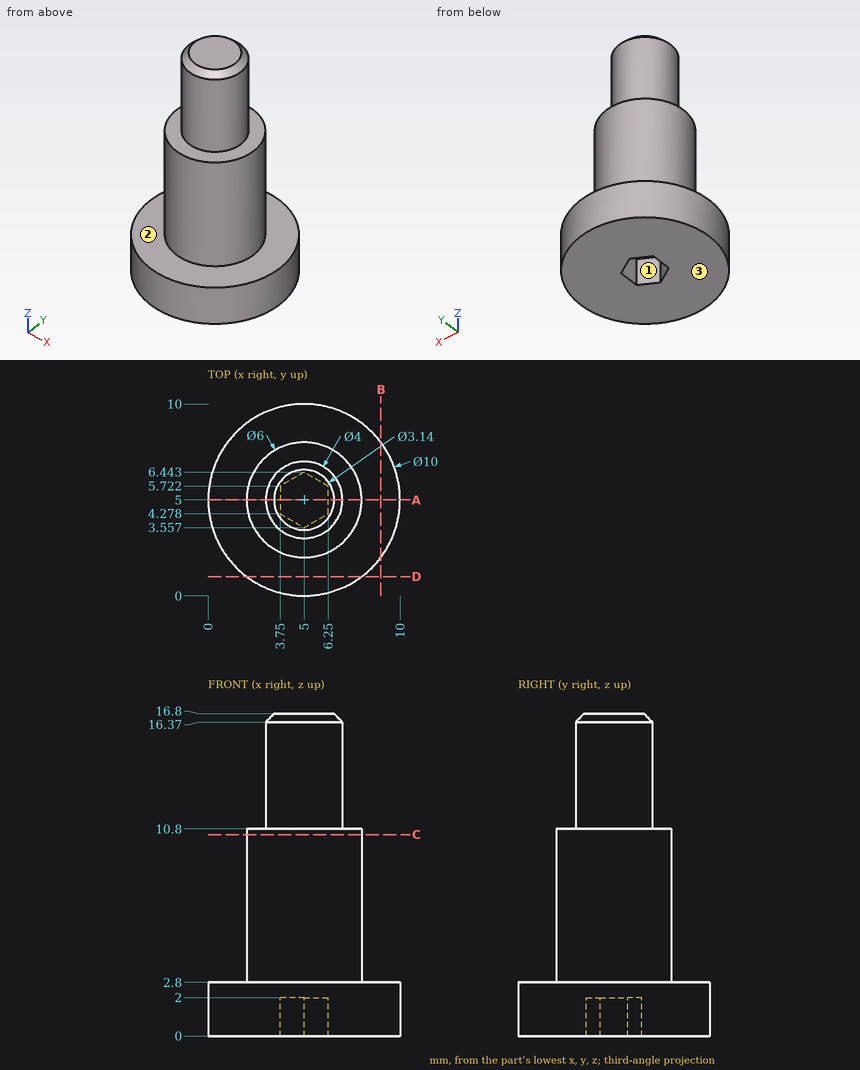
For this review, use the dimensioned drawing (mm, ordinates from the lowest corner) and the shaded views. A direction names the side the tool comes from. Coordinates: 2 decimals unless noted, no trailing zeros. Loops run counter-clockwise (first coordinate to the right, second up) from the corner with the lowest first, then second, coordinate; pieces in that order, holes last. Notation, with made-up numbers: (3.25, -23) -> (28.25, -23) arc R22 cw to (28.25, 3) -> close; hole circle Ø10 at (-40, 27.5). An arc over 180 degrees is marked (long way). Use a Markdown table: item, result. Add a question column.
1. Clearance check with flat-ended pins moving along their axes: pin 1 Ø1.2 at (y, z) = (4.5, 1) entering from +X; pin 2 Ø3 at (x, z) = (7.5, 4.5) entering from -Y; pin 3 Ø2 at (y, z) = (4, 6) entering from -X; pin 4 Ø3 at (x, z) = (7, 9.5) entering from +Y. State where each tip first meets the part, or that it passes through.
2. Add section C-C on z = 10.5. Write out the cut boundary in (x, y).
3. Add section A-A on y = 5. Write out the cut boundary in (x, z).
4. To check wall thickness, follow line 1 (Z direction, x = 1.75, y = 1.75); line 2 (Z direction, x = 5.5, y = 4); line 3 (Y direction, x = 6.75, z = 10) (1 decimal). State the ranges of each line that lie inside material, in increasing order.
5. Add section B-B on x = 9. Write out the cut boundary in (y, z).
6. Machinability: for the marked faces 1, 2 and 3, which of the approach directions +Z, -Z, +X, -X, +Y, -Y give a long, thin tool a straight path to every point of the face, cutting with its end or side? Answer none if there is none.
Returned:
| question | item | result |
|---|---|---|
| 1 | pin 1 | stops at x = 10 |
| 1 | pin 2 | stops at y = 2.17 |
| 1 | pin 3 | stops at x = 2 |
| 1 | pin 4 | stops at y = 7.96 |
| 2 | outline | circle Ø6 at (5, 5) |
| 3 | outline | (0, 0) -> (3.75, 0) -> (3.75, 2) -> (6.25, 2) -> (6.25, 0) -> (10, 0) -> (10, 2.8) -> (8, 2.8) -> (8, 10.8) -> (7, 10.8) -> (7, 16.37) -> (6.57, 16.8) -> (3.43, 16.8) -> (3, 16.37) -> (3, 10.8) -> (2, 10.8) -> (2, 2.8) -> (0, 2.8) -> close |
| 4 | line 1 | z = 0 to 2.8 |
| 4 | line 2 | z = 2 to 16.8 |
| 4 | line 3 | y = 2.6 to 7.4 |
| 5 | outline | (2, 0) -> (8, 0) -> (8, 2.8) -> (2, 2.8) -> close |
| 6 | face 1 | -Z |
| 6 | face 2 | +Z |
| 6 | face 3 | -Z, +X, -X, +Y, -Y |
